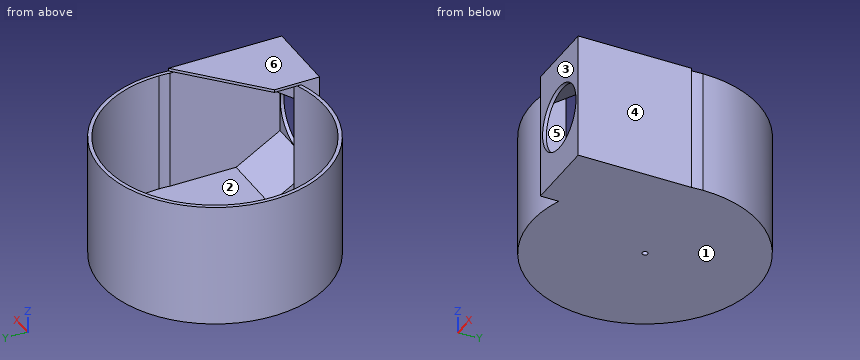
```python
from build123d import *

# Parameters (mm, degrees)
F1_DEPTH  = 279.4
F3_T      = -8.382
F4_D      = 146.05
F4_DEPTH  = 12.7
F4_TIP    = 43.8778467045
F6_DEPTH  = 147.32
F8_DEPTH  = 6.35
F10_D     = 12.7
F10_DEPTH = 12.7
F10_TIP   = 3.8154649308


with BuildPart() as f1:
    # F0 (on Top) → F1 (new body)
    with BuildSketch(Plane.XY):
        with BuildLine():
            Line((87.6268090251, -25.4), (252.7268090251, -25.4))
            ThreePointArc((252.7268090251, -25.4), (253.68150257, -12.7159448652), (254, 0))
            ThreePointArc((254, 0), (-208.2945144409, 145.3595378839), (87.6268090251, -238.4062548258))
            Line((87.6268090251, -238.4062548258), (87.6268090251, -25.4))
        make_face()
        with BuildLine():
            ThreePointArc((87.6268090251, -238.4062548258), (200.7562265004, -155.6050690733), (252.7268090251, -25.4))
            Line((252.7268090251, -25.4), (87.6268090251, -25.4))
            Line((87.6268090251, -25.4), (87.6268090251, -238.4062548258))
        make_face()
        with BuildLine():
            Line((252.7268090251, -279.4), (252.7268090251, -25.4))
            ThreePointArc((252.7268090251, -25.4), (200.7562265004, -155.6050690733), (87.6268090251, -238.4062548258))
            Line((87.6268090251, -238.4062548258), (87.6268090251, -279.4))
            Line((87.6268090251, -279.4), (252.7268090251, -279.4))
        make_face()
    extrude(amount=F1_DEPTH)

    # F3
    f3_openings = [f1.faces().sort_by_distance(p)[0] for p in [
        (15.178098, -16.804954, 279.4),
    ]]
    offset(amount=F3_T, openings=f3_openings, kind=Kind.INTERSECTION)

    # F4
    with Locations(Plane.XZ.offset(279.4)):
        with Locations((170.1768090251, 139.7)):
            Hole(F4_D / 2, depth=F4_DEPTH)
            with Locations((0, 0, -(F4_DEPTH + F4_TIP / 2))):  # 118° drill point
                Cone(0, F4_D / 2, F4_TIP, mode=Mode.SUBTRACT)

    # F5 (on face) → F6 (join)
    with BuildSketch(Plane(origin=(244.3448090251, 0, 0), x_dir=(0, -1, 0), z_dir=(-1, 0, 0))):
        Polygon((271.018, 66.548), (172.6248780656, 8.382), (271.018, 8.382), align=None)
        Polygon((271.018, 212.852), (271.018, 279.4), (178.0887059319, 279.4), align=None)
    extrude(amount=F6_DEPTH)

    # F7 (on face) → F8 (join)
    with BuildSketch(Plane.XY.offset(279.4)):
        Polygon((87.6268090251, -178.0887059319), (87.6268090251, -279.4), (252.7268090251, -279.4), (252.7268090251, -25.4), align=None)
    extrude(amount=F8_DEPTH)

    # F10
    with Locations(Plane.XY.offset(8.382)):
        with Locations((0, 0)):
            Hole(F10_D / 2, depth=F10_DEPTH)
            with Locations((0, 0, -(F10_DEPTH + F10_TIP / 2))):  # 118° drill point
                Cone(0, F10_D / 2, F10_TIP, mode=Mode.SUBTRACT)


solid = f1.part
```
The listing builds one solid part. Answer for the finished solid, in the listing's coordinates (mm). Face numbers are marked on the shaded views. A direction names the side the tool comes from. Give positions to 0.01 mm unless a question says otherwise; leave off trailing zeros. Write each loop counter-clockwise with the first axis right and the second up, starting at its lowest first coordinate (ties: lowest second). Pieces come first, ordered by that corner, then holes. Notation, with made-up numbers: (37.5, -20.5) - (70.5, -20.5) arc R22 cw to (70.5, 3.5) - close; hole circle Ø4 at (30, -23.75). An arc over 180 degrees is marked (long way). Use one line per item in the form item = value. Start each with the question number.
1) Find section A-A on x = 0. Determine the outline of the cut face in (y, z).
2) Find section C-C on y = -86. Determine the outline of the cut face in (x, z).
3) A tool of negligible diameter and unlimited length cuts with its end or side. For the marked faces 4, 5 and 6, from which of +Z, -Z, +X, -X, +Y, -Y can it reach the whole face along a straight path? Write none if from no direction.
4) Flat-ended cylindrical pins translate along their axes: pin 1 Ø8 at (x, y) = (16, -157) entering from +Z; pin 2 Ø20 at (y, z) = (-224.5, 245) entering from -X; pin 3 Ø22.5 at (y, z) = (-247.5, 171) entering from +X. Find the tip coordinate at first contact, or state that the pin passes through.
5) Find section D-D on x = -140.5. Determine the outline of the cut face in (y, z), plus the area to 3 significant figures.
6) Find section B-B on z = 258.5. Determine the outline of the cut face in (x, y), plus the area to 3 significant figures.
7) The mould has two halves that part along Y. Classify the marked faces 1, 2 and 3: pulls with the +Y half, pulls with the -Y half, needs draft (parallel to the pull), parting line crosses it, or undercut.
8) Consider line 1 along Y through (x, z) = (0, 4.25); line 2 along Y through (x, z) = (0, 207); line 3 along Z through (x, y) = (-203, 1.5). Determine where each line is inside the solid, lowest interval first. Write a range as from..to.
Geometry results:
q1.outline = (-254, 0) - (-6.35, 0) - (-6.35, 8.38) - (-245.62, 8.38) - (-245.62, 279.4) - (-254, 279.4) - close; (6.35, 0) - (254, 0) - (254, 279.4) - (245.62, 279.4) - (245.62, 8.38) - (6.35, 8.38) - close
q2.outline = (-239, 0) - (252.73, 0) - (252.73, 285.75) - (187.2, 285.75) - (187.2, 279.4) - (244.34, 279.4) - (244.34, 8.38) - (-230.07, 8.38) - (-230.07, 279.4) - (-239, 279.4) - close
q3.face_4 = +Z, -Z, +X, -Y
q3.face_5 = none
q3.face_6 = +Z, +X, -X, +Y, -Y
q4.pin_1 = 8.38
q4.pin_2 = -136.04
q4.pin_3 = 252.73
q5.outline = (-211.6, 0) - (211.6, 0) - (211.6, 279.4) - (201.46, 279.4) - (201.46, 8.38) - (-201.46, 8.38) - (-201.46, 279.4) - (-211.6, 279.4) - close
q5.area = 9,040 mm2
q6.outline = (87.63, -279.4) - (252.73, -279.4) - (252.73, -25.4) arc R254 ccw (long way) to (87.63, -238.41) - close; hole (96.01, -271.02) - (97.02, -271.02) - (97.02, -207.27) - (244.34, -207.27) - (244.34, -24.98) arc R245.62 ccw (long way) to (96.01, -226.08) - close
q6.area = 24,000 mm2
q7.face_1 = needs draft
q7.face_2 = undercut
q7.face_3 = pulls with the -Y half
q8.line_1 = -254..-6.35, 6.35..254
q8.line_2 = -254..-245.62, 245.62..254
q8.line_3 = 0..8.38
